Can you work these out from the model? Positions are in its coordinate system, mm. A direction names the side the tool comes from. Coordinates: 2 decimals unless noted, no trailing zeros. Order: outer loops, then holes, each group sorted by start corner. A loop starts at its lowest first (then second) coordinate and runs counter-clockwise, first axis right, second up. Notation, with made-up numbers: (38, 17) -> (67, 17) arc R18 cw to (67, 22) -> close; hole circle Ø9 at (-37, 26). An arc over 180 degrees is marked (long way). Answer as a JSON object with one key per item and string values. Group by question number.
(1) Which directions (+Z, -Z, +X, -X, +Y, -Y) give clear straight access to the entire face, cutting with the end or side of a thin tool? Please do faces 4 (the flat face through (44, 3, -9)), 5 (the cylindrical face through (42.5, -0.6, -12.5)), 6 (the flat face through (42, 1, -15.5)), 7 (the flat face through (6.75, 5, 2)).
(2) I want a section at A-A, the plane x = 42.5. List the corners of the cut face in (y, z) for me.
(3) I want a section at B-B, the plane x = 17.5. List the corners of the cut face in (y, z) for me.
(4) For pin 1 (4 mm diameter, centred on x = 28, y = -0.5, fed in from -Z); pin 2 (1 mm diameter, centred on y = 1.5, z = -6.5, fed in from -X); pin 3 (1 mm diameter, centred on y = -0.5, z = -9, fed in from +X); pin 4 (2 mm diameter, centred on x = 20, y = 2, fed in from -Z), each with a flat end and sliding along its axis, tell me the tip position at first contact or that it passes through.
(5) I need wall thicknesses on line 1 (Z direction, x = 28.5, y = 6); line 2 (X direction, y = -0.5, z = -11); line 3 (X direction, y = 1.5, z = -4.5). Which ranges of each line are inside material? Lowest first, please.
(6) I want a section at C-C, the plane z = -19.5. List the corners of the cut face in (x, y) for me, plus the area to 3 significant figures.
(7) If we mould it in two halves opening along Y, with no side actions, what happens to faces 1 (the flat face through (2.2, -0.2, -4.75)), 2 (the flat face through (22, 3.8, 2)), 3 (the cylindrical face through (-1.215, -0.899, -16.412))? For each: pulls with the +Y half, pulls with the -Y half, needs draft (parallel to the pull), parting line crosses it, or undercut.
from build123d import *

# Parameters (mm, degrees)
SKETCH1_W                = 47
SKETCH1_H                = 21.5
SKETCH1_W_2              = 44
SKETCH1_H_2              = 18.5
EXTRUDE_THIN1_DEPTH      = 7
SKETCH2_W                = 47
SKETCH2_H                = 21.5
BOSS_EXTRUDE1_DEPTH      = 1.2
SKETCH3_W                = 21
SKETCH3_H                = 9
CUT_EXTRUDE1_DEPTH       = 9.2
CUT_EXTRUDE2_DEPTH       = 9.2
SKETCH5_W                = 44
SKETCH5_H                = 18.5
BOSS_EXTRUDE2_DEPTH      = 1.2
SKETCH6_W                = 44
SKETCH6_H                = 12.5
CUT_EXTRUDE3_DEPTH       = 1.2
SKETCH9_W                = 42.5
SKETCH9_H                = 18.5
CUT_EXTRUDE4_DEPTH       = 3
BOSS_EXTRUDE3_DEPTH      = 15
BOSS_EXTRUDE3_DEPTH_BACK = 15
SKETCH13_W               = 3
SKETCH13_H               = 3
BOSS_EXTRUDE4_DEPTH      = 2.5
FILLET1_R                = 1
FILLET2_R                = 1


with BuildPart() as part:
    # Sketch1 → Extrude-Thin1 (new body)
    with BuildSketch(Plane(origin=(0, 0, 0), x_dir=(1, 0, 0), z_dir=(0, 1, 0))):
        with Locations((22, 9.25)):
            Rectangle(SKETCH1_W, SKETCH1_H)
        with Locations((22, 9.25)):
            Rectangle(SKETCH1_W_2, SKETCH1_H_2, mode=Mode.SUBTRACT)
    extrude(amount=EXTRUDE_THIN1_DEPTH)

    # Sketch2 → Boss-Extrude1 (add)
    with BuildSketch(Plane.XZ):
        with Locations((22, -9.25)):
            Rectangle(SKETCH2_W, SKETCH2_H)
    extrude(amount=BOSS_EXTRUDE1_DEPTH)

    # Sketch3 → Cut-Extrude1 (cut, through all)
    with BuildSketch(Plane.XZ.offset(1.2)):
        with Locations((-1.5, -9.25)):
            Rectangle(SKETCH3_W, SKETCH3_H)
    extrude(amount=-CUT_EXTRUDE1_DEPTH, mode=Mode.SUBTRACT)

    # Sketch4 → Cut-Extrude2 (cut, through all)
    with BuildSketch(Plane.XZ.offset(1.2)):
        with BuildLine():
            Line((25.25, -11.25), (25.25, -7.25))
            ThreePointArc((25.25, -7.25), (26.5, -6), (27.75, -7.25))
            Line((27.75, -7.25), (27.75, -11.25))
            ThreePointArc((27.75, -11.25), (26.5, -12.5), (25.25, -11.25))
        make_face()
        with BuildLine():
            Line((43.75, -11.25), (43.75, -7.25))
            ThreePointArc((43.75, -7.25), (42.5, -6), (41.25, -7.25))
            Line((41.25, -7.25), (41.25, -11.25))
            ThreePointArc((41.25, -11.25), (42.5, -12.5), (43.75, -11.25))
        make_face()
    extrude(amount=-CUT_EXTRUDE2_DEPTH, mode=Mode.SUBTRACT)

    # Sketch5 → Boss-Extrude2 (add)
    with BuildSketch(Plane(origin=(0, 5.5, 0), x_dir=(-1, 0, 0), z_dir=(0, -1, 0))):
        with Locations((-22, 9.25)):
            Rectangle(SKETCH5_W, SKETCH5_H)
    extrude(amount=BOSS_EXTRUDE2_DEPTH)

    # Sketch6 → Cut-Extrude3 (cut)
    with BuildSketch(Plane(origin=(0, 4.3, 0), x_dir=(-1, 0, 0), z_dir=(0, -1, 0))):
        with Locations((-22, 9.25)):
            Rectangle(SKETCH6_W, SKETCH6_H)
    extrude(amount=-CUT_EXTRUDE3_DEPTH, mode=Mode.SUBTRACT)

    # Sketch9 → Cut-Extrude4 (cut)
    with BuildSketch(Plane(origin=(0, 5.5, 0), x_dir=(1, 0, 0), z_dir=(0, 1, 0))):
        with Locations((22, 9.25)):
            Rectangle(SKETCH9_W, SKETCH9_H)
    extrude(amount=-CUT_EXTRUDE4_DEPTH, mode=Mode.SUBTRACT)

    # Sketch10 → Boss-Extrude3 (add, two sides)
    with BuildSketch(Plane.ZY.offset(-21.75)) as boss_extrude3_sk:
        Polygon((-20, 2.8), (-21, 3.8), (-20, 3.8), align=None)
        Polygon((2.5, 3.8), (1.5, 3.8), (1.5, 2.8), align=None)
        Polygon((1.5, 5.8), (2.5, 4.8), (1.5, 4.8), align=None)
        Polygon((-21, 4.8), (-20, 4.8), (-20, 5.8), align=None)
    extrude(amount=BOSS_EXTRUDE3_DEPTH)
    extrude(boss_extrude3_sk.sketch, amount=-BOSS_EXTRUDE3_DEPTH_BACK)

    # Sketch13 → Boss-Extrude4 (add)
    with BuildSketch(Plane(origin=(0, 0, 0), x_dir=(1, 0, 0), z_dir=(0, 1, 0))):
        with Locations((1.5, 1.5)):
            Rectangle(SKETCH13_W, SKETCH13_H)
        with Locations((42.5, 17)):
            Rectangle(SKETCH13_W, SKETCH13_H)
        with Locations((42.5, 1.5)):
            Rectangle(SKETCH13_W, SKETCH13_H)
        with Locations((1.5, 17)):
            Rectangle(SKETCH13_W, SKETCH13_H)
    extrude(amount=BOSS_EXTRUDE4_DEPTH)

    # Fillet1
    fillet1_edges = [part.edges().sort_by_distance(p)[0] for p in [
        (-1.5, 2.9, -20),
        (45.5, 2.9, -20),
        (45.5, 2.9, 1.5),
        (-1.5, 2.9, 1.5),
    ]]
    fillet(fillet1_edges, radius=FILLET1_R)

    # Fillet2
    fillet2_edges = [part.edges().sort_by_distance(p)[0] for p in [
        (22, -1.2, -20),
        (45.5, -1.2, -9.25),
        (22, -1.2, 1.5),
        (-1.5, -1.2, -2.125),
        (-1.207106781, -1.2, 1.207106781),
        (45.207106781, -1.2, 1.207106781),
        (45.207106781, -1.2, -19.707106781),
        (-1.207106781, -1.2, -19.707106781),
        (-1.5, -1.2, -16.375),
    ]]
    fillet(fillet2_edges, radius=FILLET2_R)


solid = part.part
Computed values:
{
 "1": {"face 4": "none", "face 5": "+Y, -Y", "face 6": "+Y", "face 7": "+Z, -X, +Y, -Y"},
 "2": {"outline": "(-1.2, -19) arc R1 ccw to (-0.2, -20) -> (7, -20) -> (7, -18.5) -> (2.5, -18.5) -> (2.5, -15.5) -> (0, -15.5) -> (0, -12.5) -> (-1.2, -12.5) -> close; (-1.2, -6) -> (0, -6) -> (0, -3) -> (2.5, -3) -> (2.5, 0) -> (7, 0) -> (7, 1.5) -> (-0.2, 1.5) arc R1 ccw to (-1.2, 0.5) -> close"},
 "3": {"outline": "(-1.2, -19) arc R1 ccw to (-0.2, -20) -> (2.8, -20) -> (3.8, -21) -> (3.8, -20) -> (4.8, -20) -> (4.8, -21) -> (5.8, -20) -> (7, -20) -> (7, -18.5) -> (0, -18.5) -> (0, 0) -> (7, 0) -> (7, 1.5) -> (5.8, 1.5) -> (4.8, 2.5) -> (4.8, 1.5) -> (3.8, 1.5) -> (3.8, 2.5) -> (2.8, 1.5) -> (-0.2, 1.5) arc R1 ccw to (-1.2, 0.5) -> close"},
 "4": {"pin 1": "stops at z = -20", "pin 2": "stops at x = 44", "pin 3": "stops at x = 45.5", "pin 4": "stops at z = -20.2"},
 "5": {"line 1": "z = -20 to -18.5, 0 to 1.5", "line 2": "x = 9 to 25.25, 27.75 to 41.25, 43.75 to 45.45", "line 3": "x = -1.5 to 0, 44 to 45.5"},
 "6": {"outline": "(-1.37, -0.2) arc R0.87 ccw to (-0.5, -1.07) -> (44.5, -1.07) arc R0.87 ccw to (45.37, -0.2) -> (45.37, 7) -> (-1.37, 7) -> close", "area": "377 mm2"},
 "7": {"face 1": "needs draft", "face 2": "undercut", "face 3": "pulls with the -Y half"}
}
